Autodesk Inventor part; units mm, degrees
ref_plane "YZ Plane" through (0, 0, 0) normal (1, 0, 0) x (0, 1, 0)
ref_plane "XZ Plane" through (0, 0, 0) normal (0, 1, 0) x (-1, 0, 0)
ref_plane "XY Plane" through (0, 0, 0) normal (0, 0, 1) x (1, 0, 0)
sketch "Sketch1" plane through (0, 0, 0) normal (0, 0, 1) x (1, 0, 0)
  line L0 (0, -103.3729) -> (0, 23.6271) construction
  line L1 (-12.446, -103.3729) -> (-12.446, 23.6271)
  line L2 (12.446, 23.6271) -> (12.446, -103.3729)
  arc A0 (-12.446, -103.3729) -> (12.446, -103.3729) centre (0, -103.3729) ccw
  arc A1 (12.446, 23.6271) -> (-12.446, 23.6271) centre (0, 23.6271) ccw
  point P0 (0, 0)
  point P1 (0, -39.8729)
  dimension "d0" = 63.5
  dimension "d1" = 24.892
extrude "Extrusion1" add sketch "Sketch1" along normal blind 6.096
sketch "Sketch2" plane through (0, 0, 6.096) normal (0, 0, 1) x (1, 0, 0)
  line L0 (-12.446, 23.6271) -> (-12.446, -103.3729)
  arc A0 (-12.446, -103.3729) -> (12.446, -103.3729) centre (0, -103.3729) ccw
  line L1 (12.446, -103.3729) -> (12.446, 23.6271)
  arc A1 (12.446, 23.6271) -> (-12.446, 23.6271) centre (0, 23.6271) ccw
  point P0 (0, 0)
  point P1 (0, -39.8729)
hole "Hole1" at (0, 23.6271, 6.096) at (0, -103.3729, 6.096) direction (0, 0, -1) diameter 12.446 depth 5.7785 tip angle 118
hole "Hole2" at (0, -39.8729, 0) direction (0, 0, 1) diameter 5.08 depth 5.7785 tip angle 118
sketch "Sketch3" plane through (0, 0, 0) normal (0, 0, -1) x (-1, 0, 0)
  circle A0 centre (0, -39.8729) radius 2.0116
  arc A1 (10, -39.8729) -> (-10, -39.8729) centre (0, -39.8729) ccw construction
  arc A2 (12.032, -39.8729) -> (-12.032, -39.8729) centre (0, -39.8729) ccw
  arc A3 (7.968, -39.8729) -> (-7.968, -39.8729) centre (0, -39.8729) ccw
  arc A4 (7.968, -39.8729) -> (12.032, -39.8729) centre (10, -39.8729) ccw
  arc A5 (-12.032, -39.8729) -> (-7.968, -39.8729) centre (-10, -39.8729) ccw
  point P0 (0, 0)
  dimension "d18" = 2.032
  dimension "d19" = 10
extrude "Extrusion2" cut sketch "Sketch3" against normal through all contours A4 A3 A5 A2
sketch "Sketch4" plane through (12.446, -103.3729, 0) normal (1, 0, 0) x (0, 0, -1)
  line L0 (0, 0) -> (0, 127)
  line L1 (0, 127) -> (-6.096, 127)
  line L2 (-6.096, 0) -> (-6.096, 127)
  line L3 (0, 0) -> (-6.096, 0)
  point P0 (0, 103.3729)
extrude "Extrusion3" add sketch "Sketch4" along normal blind 31.75
sketch "Sketch5" plane through (0, 0, 0) normal (0, 0, -1) x (-1, 0, 0)
  line L0 (-23.4086, 4.8323) -> (-58.9686, 4.8323)
  line L1 (-58.9686, 4.8323) -> (-58.9686, 40.3923)
  line L2 (-58.9686, 40.3923) -> (-23.4086, 40.3923)
  line L3 (-23.4086, 40.3923) -> (-23.4086, 4.8323)
  circle A0 centre (-41.1886, 22.6123) radius 12.7
  line L4 (8.5245, 22.6123) -> (-42.691, 22.6123)
  line L5 (-12.446, 23.6271) -> (-44.196, 23.6271)
  circle A1 centre (0, 23.6271) radius 5.6946
  point P0 (0, 0)
  point P1 (-29.3576, 32.6261)
  point P2 (-43.9453, 37.8652)
  point P3 (-55.7764, 27.8514)
  point P4 (-53.0197, 12.5985)
  point P5 (-38.432, 7.3594)
  point P6 (-26.6009, 17.3732)
  point P7 (-47.5832, 13.0873)
  point P8 (-42.5032, 13.0873)
  point P9 (-28.4886, 22.6123)
  point P10 (-23.4086, 22.6123)
  dimension "d24" = 35.56
  dimension "d25" = 35.56
  dimension "d26" = 25.4
  dimension "d27" = 17.78
  dimension "d28" = 17.78
  dimension "d29" = 15.5
  dimension "d32" = 360
  dimension "d45" = 41.1886
extrude "Extrusion4" add sketch "Sketch5" against normal up to surface (6.096 mm away) contours L0 L1 L2 L3 L5 A0 L4 | L4 A0 L5 L3 | A0
extrude "Extrusion5" cut sketch "Sketch5" against normal through all contours A0
hole "Hole3" at (26.6009, 17.3732, 0) at (38.432, 7.3594, 0) at (53.0197, 12.5985, 0) at (55.7764, 27.8514, 0) at (43.9453, 37.8652, 0) at (29.3576, 32.6261, 0) direction (0, 0, 1) diameter 2.3368 depth 5.7785 tip angle 118
equation "\"d27\" = 0.5 * d25"
equation "\"d28\" = 0.5 * d24"
properties part number "new conveyor bar"
Source: CAD feature listing. Evaluate the final solid. Frame: model axes, mm. A direction names the side the tool comes from. Coordinates: 2 decimals unless noted, no trailing zeros. Loops run counter-clockwise (first coordinate to the right, second up) from the corner with the lowest first, then second, coordinate; pieces in that order, holes last. Notation, with made-up numbers: (25.25, 46) - (72.25, 46) arc R25 cw to (72.25, 60) - close; hole circle Ø4 at (39.25, -38.5). An arc over 180 degrees is marked (long way). Return JSON: item names as keys, results as strings.
Q1. Section A-A, the plane x = 49. Return loops of the section in (y, z), plus the area to 3 significant figures.
Results:
{"outline": "(4.83, 0) - (12.6, 0) - (12.6, 6.1) - (4.83, 6.1) - close; (32.63, 0) - (40.39, 0) - (40.39, 6.1) - (32.63, 6.1) - close", "area": "94.7 mm2"}
Q2. Contact query for flat-ended pins moving along their axis: P1, Ø1.5, axis at x = 11.5, z = 4, coming from the +Y side; P2, Ø3, axis at x = 2.5, z = 3, coming from the -Y side; P3, Ø11, axis at x = 0, y = 23.63, coming from the +Z side; P4, Ø1.8, axis at y = 35, z = 2, coming from the -X side. Output: stop coordinate, or through.
Results:
{"P1": "y = 29.9", "P2": "y = -115.78", "P3": "through", "P4": "x = -6.72"}
Q3. Section B-B, the plane x = 0. Return loops of the section in (y, z), plus the area to 3 significant figures.
Results:
{"outline": "(-115.82, 0) - (-109.07, 0) - (-109.6, 0.32) - (-109.6, 6.1) - (-115.82, 6.1) - close; (-97.68, 0) - (-42.41, 0) - (-42.41, 5.78) - (-41.88, 6.1) - (-97.15, 6.1) - (-97.15, 0.32) - close; (-37.86, 6.1) - (-37.33, 5.78) - (-37.33, 0) - (-31.9, 0) - (-31.9, 6.1) - close; (-27.84, 0) - (17.93, 0) - (17.4, 0.32) - (17.4, 6.1) - (-27.84, 6.1) - close; (29.32, 0) - (36.07, 0) - (36.07, 6.1) - (29.85, 6.1) - (29.85, 0.32) - close", "area": "719 mm2"}
Q4. Access query for faces 5 (the flat face through (51, 4.832, 3)), 6 (the cylindrical face through (-0.76, -37.45, 2.93)), 7 (the cylindrical face through (-0.274, -97.156, 3.166)), 8 (the cylindrical face through (-0.175, -31.907, 3.005)). Directions: +Z, -Z, +X, -X, +Y, -Y. A direction counts if a zero-diameter tool reaches every point of the face in a straight line with its end or side. Return the directions, or none.
Results:
{"face 5": "+Z, -Z, +X, -Y", "face 6": "-Z", "face 7": "+Z", "face 8": "+Z, -Z"}
Q5. Section C-C, the plane z = 2. Give the number of separate pieces and of enclosed holes in the cut face, plus the area to 3 significant figures.
Results:
{"separate pieces": "1", "enclosed holes": "11", "area": "7,620 mm2"}
Q6. Material intervals for line 1 along Y through (x, z) = (0, 4.9); line 2 along Y through (x, z) = (2, 1); line 3 along X through (y, z) = (-61, 4.25), sorted ascending.
Results:
{"line 1": "-115.82 to -109.6, -97.15 to -42.41, -37.33 to -31.9, -27.84 to 17.4, 29.85 to 36.07", "line 2": "-115.66 to -109.27, -97.48 to -41.44, -38.31 to -32.16, -28.01 to 17.73, 29.52 to 35.91", "line 3": "-12.45 to 44.2"}
Q7. Section D-D, the plane y = -8. Return loops of the section in (x, z), plus the area to 3 significant figures.
Results:
{"outline": "(-12.45, 0) - (44.2, 0) - (44.2, 6.1) - (-12.45, 6.1) - close", "area": "345 mm2"}
Q8. Mould query, pull axis Y, two halves, no side actions, for faces 1 (the cylindrical face through (-9.955, -41.904, 3.005)), 2 (the flat face through (28, -103.373, 3)), 3 (the flat face through (23.409, 32, 3)), 4 (the flat face through (18, 23.627, 3)). Classes: released by +Y, released by -Y, zero draft, split by the parting line, or undercut.
Results:
{"face 1": "undercut", "face 2": "released by -Y", "face 3": "zero draft", "face 4": "released by +Y"}
